The model under review builds one solid part; all positions refer to its coordinate system, in mm. Face numbers are marked on the shaded views. Give positions to 0.01 mm unless a question says otherwise; leave off trailing zeros. Order: outer loops, then holes, each group sorted by start corner. A loop starts at its lowest first (then second) coordinate and runs counter-clockwise, first axis right, second up. Notation, with made-up numbers: (-30, -32) - (-16, -32) arc R27 ccw to (-16, -6) - close; hole circle Ø10 at (-22.5, -17). An arc over 180 degrees is marked (long way). Write item = value, one per line. Start each with the question number.
1. For P1, Ø4, axis at y = 33.5, z = -1.5, coming from the -X side; P2, Ø2, axis at x = 23.5, z = -10.5, coming from the +Y side; P3, Ø4, axis at y = 32.5, z = 4.5, coming from the +X side, all flat-tipped, find the tip position at first contact; note any pin that passes through.
2. Mouldability with a two-part tool opening along X and no side actions: class the marked faces 1, 2, 3 and 4 as pulls with the +X half, pulls with the -X half, needs draft (parallel to the pull), parting line crosses it, or undercut.
3. We need section A-A, the plane y = 51. Give the boundary of the cut face in (x, z).
4. Wall thickness on probe 1 along X at (y, z) = (46, -9); probe 2 along Y at (x, z) = (40, -25): over which ranges is each line inside the solid? List them lowest first.
5. We need section B-B, the plane z = 9. Give the boundary of the cut face in (x, y), and give its area (3 significant figures).
6. We need section C-C, the plane x = 20. Give the boundary of the cut face in (y, z).
from build123d import *

# Parameters (mm, degrees)
SKETCH1_W           = 72.370080969
SKETCH1_H           = 78.237925372
BOSS_EXTRUDE1_DEPTH = 7.874
BOSS_EXTRUDE3_DEPTH = 68.58


with BuildPart() as part:
    # Sketch1 → Boss-Extrude1 (new body)
    with BuildSketch(Plane(origin=(0, 0, 0), x_dir=(1, 0, 0), z_dir=(0, 1, 0))):
        with Locations((17.407938396, 20.928645037)):
            Rectangle(SKETCH1_W, SKETCH1_H)
    extrude(amount=BOSS_EXTRUDE1_DEPTH)

    # Sketch2 → Boss-Extrude3 (add)
    with BuildSketch(Plane(origin=(0, 7.874, 0), x_dir=(1, 0, 0), z_dir=(0, 1, 0))):
        Polygon((41.192023567, 60.047607723), (41.192023567, 20.928645037), (41.192023567, -18.190317649), (45.917338502, -18.190317649), (45.917338502, 60.047607723), align=None)
        Polygon((-6.376146777, -18.190317649), (-6.376146777, 20.928645037), (-6.376146777, 60.047607723), (-11.101461711, 60.047607723), (-11.101461711, -18.190317649), align=None)
    extrude(amount=BOSS_EXTRUDE3_DEPTH)


solid = part.part
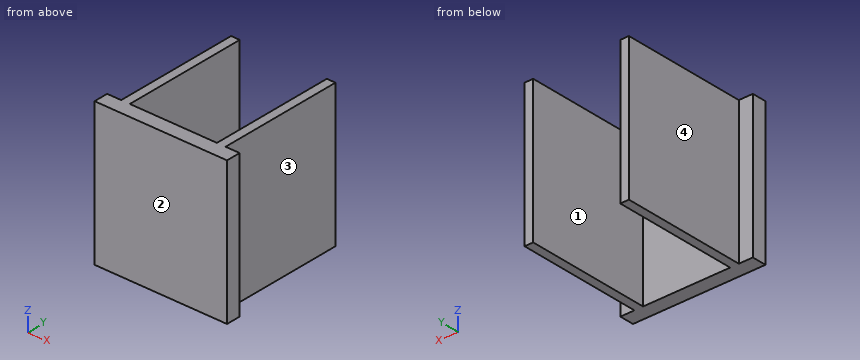
Model answer:
q1.P1 = -11.1
q1.P2 = 7.87
q1.P3 = 45.92
q2.face_1 = undercut
q2.face_2 = needs draft
q2.face_3 = pulls with the +X half
q2.face_4 = pulls with the -X half
q3.outline = (-11.1, -60.05) - (-6.38, -60.05) - (-6.38, 18.19) - (-11.1, 18.19) - close; (41.19, -60.05) - (45.92, -60.05) - (45.92, 18.19) - (41.19, 18.19) - close
q4.probe_1 = -11.1 to -6.38, 41.19 to 45.92
q4.probe_2 = 0 to 7.87
q5.outline = (-18.78, 0) - (53.59, 0) - (53.59, 7.87) - (45.92, 7.87) - (45.92, 76.45) - (41.19, 76.45) - (41.19, 7.87) - (-6.38, 7.87) - (-6.38, 76.45) - (-11.1, 76.45) - (-11.1, 7.87) - (-18.78, 7.87) - close
q5.area = 1,220 mm2
q6.outline = (0, -60.05) - (7.87, -60.05) - (7.87, 18.19) - (0, 18.19) - close
